For this review, take the finished solid that the model builds, in its own axes (mm). Face numbers are marked on the shaded views. A direction names the side the tool comes from. Round coordinates to 2 decimals unless told otherwise and drop trailing zeros. Write each loop counter-clockwise with the first axis right and the second up, starting at its lowest first coordinate (ties: lowest second). Pieces come first, ordered by that corner, then holes. Notation, with made-up numbers: (-10, -17) - (48, -17) arc R12 ccw to (48, 2) - close; hole circle Ø3 at (45.5, 14.25). An arc over 180 degrees is marked (long way). One line per item, written item: value. Start each with the question number.
Q1. For probe 1 along Y at (x, z) = (-1, 4.5); probe 2 along X at (y, z) = (-0.5, -12.5); probe 3 along X at (y, z) = (-6, 0), list the stretches that pass through material, from the lowest coordinate up.
Q2. Mouldability with a two-part tool opening along Z and no side actions: class the marked faces 1, 2 and 3 as +Z half, -Z half, draft (parallel to the pull), parting line (faces both ways), or undercut.
Q3. Add section A-A on y = -9.5. Write out the cut boundary in (x, z).
Q4. Add section B-B on x = 0. Write out the cut boundary in (y, z).
Q5. Tool access review of the marked faces 4, 5, 6, 7 and 8: name each direction out of +Z, -Z, +X, -X, +Y, -Y from which nothing blocks a thin tool from reaching the whole face with its end or side.
Q6. Add section C-C on y = 0. Give the number of separate pieces and of enclosed holes in the cut face, and give its area (3 significant figures).
Q7. Clearance check with flat-ended pins moving along their axes: pin 1 Ø10 at (y, z) = (-7, 2.5) entering from -X; pin 2 Ø14 at (x, z) = (-5, 11.5) entering from +Y; pin 3 Ø1 at (x, y) = (-1, 5) entering from -Z; pin 4 Ø1 at (y, z) = (-8, 6.5) entering from +X. State where each tip first meets the part, or that it passes through.
```python
from build123d import *

# Parameters (mm, degrees)
FUROS_GUIA_COM_4_0MM2_D            = 4
FUROS_GUIA_COM_4_0MM1_REACH        = 51.881
FUROS_GUIA_COM_4_0MM1_BORE_R       = 2
ESBO_O7_W                          = 18
ESBO_O7_H                          = 6
CORTE_EXTRUS_O4_DEPTH              = 2
ESBO_O11_R                         = 3
REBAIXO_1_DEPTH                    = 2
ESBO_O13_R                         = 3
REBAIXO_2_DEPTH                    = 4
ESBO_O14_W                         = 21
ESBO_O14_H                         = 8
CORTE_EXTRUS_O8_DEPTH              = 2
ESBO_O15_W                         = 21
ESBO_O15_H                         = 8
ESBO_O15_R                         = 3
CORTE_EXTRUS_O13_DEPTH             = 2
CORTE_EXTRUS_O14_START             = -15
CORTE_EXTRUS_O14_DEPTH             = 21
ESBO_O18_R                         = 3
CORTE_EXTRUS_O15_DEPTH             = 4
CORTE_EXTRUS_O16_REACH             = 34.016
CORTE_EXTRUS_O16_DIRECTION_2_DEPTH = 6


with BuildPart() as part:
    # Esbo_o1 → Revolu_o1 (revolve)
    with BuildSketch(Plane.XY, mode=Mode.PRIVATE) as revolu_o1_sk:
        Polygon((0, -15), (20, -15), (20, 5), (19.5, 5), (19.5, 6), (20, 6.5), (20, 10.5), (19.5, 11), (15, 11), (15, -9), (3.5, -9), (3.5, -12.5), (0, -12.5), align=None)
    revolve(revolu_o1_sk.sketch.rotate(Axis((0, 0, 0), (0, 1, 0)), 90), axis=Axis((0, 0, 0), (0, 1, 0)))

    # Furos-guia com _4.0mm2 (through all)
    with Locations(Plane(origin=(-20, 0, 0), x_dir=(0, 0, -1), z_dir=(-1, 0, 0))):
        with Locations((0, 0)):
            Hole(FUROS_GUIA_COM_4_0MM2_D / 2)

    # Furos-guia com _4.0mm1 bore (on position points) → Furos-guia com _4.0mm1 (cut, up to next)
    with BuildSketch(Plane(origin=(-18.126155741, 0, -8.452365235), x_dir=(0.422618261741, 0, -0.906307787037), z_dir=(-0.906307787037, 0, -0.422618261741)), mode=Mode.PRIVATE) as furos_guia_com_4_0mm1_sk1:
        Circle(FUROS_GUIA_COM_4_0MM1_BORE_R)
    furos_guia_com_4_0mm1_tool1 = extrude(furos_guia_com_4_0mm1_sk1.sketch, amount=-FUROS_GUIA_COM_4_0MM1_REACH, mode=Mode.PRIVATE) & part.part
    add(furos_guia_com_4_0mm1_tool1.solids().sort_by_distance((-18.126156, 0, -8.452365))[0], mode=Mode.SUBTRACT)

    # Esbo_o7 → Corte-extrus_o4 (cut)
    with BuildSketch(Plane(origin=(20, 0, 0), x_dir=(0, -1, 0), z_dir=(1, 0, 0))):
        with Locations((6, 0)):
            Rectangle(ESBO_O7_W, ESBO_O7_H)
    extrude(amount=-CORTE_EXTRUS_O4_DEPTH, mode=Mode.SUBTRACT)

    # Esbo_o11 → Rebaixo 1 (cut)
    with BuildSketch(Plane(origin=(18, 0, 0), x_dir=(0, 0, -1), z_dir=(1, 0, 0))):
        Circle(ESBO_O11_R)
    extrude(amount=-REBAIXO_1_DEPTH, mode=Mode.SUBTRACT)

    # Esbo_o13 → Rebaixo 2 (cut)
    with BuildSketch(Plane(origin=(-18.126155741, 0, -8.452365235), x_dir=(0, -1, 0), z_dir=(-0.9063077870366467, 0, -0.4226182617407065))):
        with Locations(Location((0, 0, 0), (0, 0, 90))):
            Circle(ESBO_O13_R)
    extrude(amount=-REBAIXO_2_DEPTH, mode=Mode.SUBTRACT)

    # Esbo_o14 → Corte-extrus_o8 (cut)
    with BuildSketch(Plane(origin=(-18.126155741, 0, -8.452365235), x_dir=(0, -1, 0), z_dir=(-0.9063077870366467, 0, -0.4226182617407065))):
        with Locations((4.5, 0)):
            Rectangle(ESBO_O14_W, ESBO_O14_H)
    extrude(amount=-CORTE_EXTRUS_O8_DEPTH, mode=Mode.SUBTRACT)

    # Esbo_o15 → Corte-extrus_o13 (cut)
    with BuildSketch(Plane(origin=(-20, 0, 0), x_dir=(0, -1, 0), z_dir=(-1, 0, 0))):
        with Locations((4.5, 0)):
            Rectangle(ESBO_O15_W, ESBO_O15_H)
        with Locations(Location((0, 0, 0), (0, 0, 270))):
            Circle(ESBO_O15_R, mode=Mode.SUBTRACT)
    extrude(amount=-CORTE_EXTRUS_O13_DEPTH, mode=Mode.SUBTRACT)

    # Esbo_o17 → Corte-extrus_o14 (cut)
    with BuildSketch(Plane(origin=(0, 0, 0), x_dir=(1, 0, 0), z_dir=(0, 1, 0)).offset(CORTE_EXTRUS_O14_START)):
        with BuildLine():
            Line((-18, 3.990503928), (-18, -8.717797887))
            ThreePointArc((-18, -8.717797887), (-19.525920142, 4.328792279), (-12.629239577, 15.508136822))
            Line((-12.629239577, 15.508136822), (-18, 3.990503928))
        make_face()
    extrude(amount=CORTE_EXTRUS_O14_DEPTH, mode=Mode.SUBTRACT)

    # Esbo_o18 → Corte-extrus_o15 (cut)
    with BuildSketch(Plane(origin=(-20, 0, 0), x_dir=(0, -1, 0), z_dir=(-1, 0, 0))):
        with Locations(Location((0, 0, 0), (0, 0, 270))):
            Circle(ESBO_O18_R)
    extrude(amount=-CORTE_EXTRUS_O15_DEPTH, mode=Mode.SUBTRACT)

    # Esbo_o9 → Corte-extrus_o16 (cut, up to next)
    with BuildSketch(Plane(origin=(0, 0, 0), x_dir=(1, 0, 0), z_dir=(0, 1, 0)), mode=Mode.PRIVATE) as corte_extrus_o16_sk1:
        with BuildLine():
            Line((16.845642244, 10.780739186), (16.845642244, -10.780739186))
            ThreePointArc((16.845642244, -10.780739186), (20, 0), (16.845642244, 10.780739186))
        make_face()
    corte_extrus_o16_tool1 = extrude(corte_extrus_o16_sk1.sketch, amount=-CORTE_EXTRUS_O16_REACH, mode=Mode.PRIVATE) & part.part
    add(corte_extrus_o16_tool1.solids().sort_by_distance((18.116323, 0, 0))[0], mode=Mode.SUBTRACT)

    # Esbo_o9 → Corte-extrus_o16 direction 2 (cut)
    with BuildSketch(Plane(origin=(0, 0, 0), x_dir=(1, 0, 0), z_dir=(0, 1, 0))):
        with BuildLine():
            Line((16.845642244, 10.780739186), (16.845642244, -10.780739186))
            ThreePointArc((16.845642244, -10.780739186), (20, 0), (16.845642244, 10.780739186))
        make_face()
    extrude(amount=CORTE_EXTRUS_O16_DIRECTION_2_DEPTH, mode=Mode.SUBTRACT)


solid = part.part
```
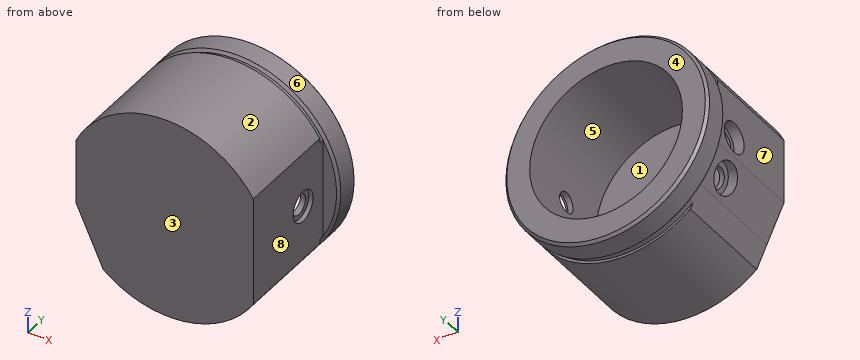
Result set:
1. probe 1: y = -15 to -9
1. probe 2: x = -14.03 to -8.29, 8.29 to 15.61
1. probe 3: x = -18 to -15, 15 to 16.85
2. face 1: undercut
2. face 2: +Z half
2. face 3: draft
3. outline: (-18, -3.99) - (-12.63, -15.51) arc R20 ccw to (16.85, -10.78) - (16.85, 10.78) arc R20 ccw to (-18, 8.72) - close; hole circle Ø7 at (0, 0)
4. outline: (-15, -20) - (5, -20) - (5, -19.5) - (6, -19.5) - (6.5, -20) - (10.5, -20) - (11, -19.5) - (11, -15) - (-9, -15) - (-9, -3.5) - (-12.5, -3.5) - (-12.5, 3.5) - (-9, 3.5) - (-9, 15) - (11, 15) - (11, 19.5) - (10.5, 20) - (6.5, 20) - (6, 19.5) - (5, 19.5) - (5, 20) - (-15, 20) - close
5. face 4: +Z, -Z, +X, -X, +Y
5. face 5: +Y
5. face 6: +Y, -Y
5. face 7: +Z, -Z, -X, -Y
5. face 8: +Z, -Z, +X, -Y
6. separate pieces: 3
6. enclosed holes: 0
6. area: 423 mm^2
7. pin 1: stops at x = -18
7. pin 2: stops at y = 11
7. pin 3: stops at z = -19.99
7. pin 4: stops at x = 16.85
